The model under review builds one solid part; all positions refer to its coordinate system, in mm. Face numbers are marked on the shaded views. A direction names the side the tool comes from. Coordinates: 2 decimals unless noted, no trailing zeros. Order: outer loops, then holes, each group sorted by start corner. A loop starts at its lowest first (then second) coordinate and runs counter-clockwise, first axis right, second up. Notation, with made-up numbers: (-17, 74.25) -> (-11, 74.25) arc R18 cw to (-11, 92.25) -> close; hole circle Ø9 at (55, 6). An arc over 180 degrees is marked (long way). Put each result on its own line as item: value.
Autodesk Inventor part; units mm, degrees
ref_plane "XZ Plane" through (0, 0, 0) normal (0, 1, 0) x (-1, 0, 0)
sketch "Sketch1" plane through (0, 0, 0) normal (0, 1, 0) x (-1, 0, 0)
  line L0 (50.8, 50.8) -> (-50.8, 50.8)
  line L1 (-50.8, 50.8) -> (-50.8, -50.8)
  line L2 (-50.8, -50.8) -> (50.8, -50.8)
  line L3 (50.8, -50.8) -> (50.8, 50.8)
  line L4 (50.8, 50.8) -> (-50.8, -50.8) construction
  line L5 (-50.8, 50.8) -> (50.8, -50.8) construction
  point P0 (0, 0)
  dimension "d0" = 101.6
  dimension "d1" = 101.6
extrude "Extrusion1" add sketch "Sketch1" along normal blind 6.35
sketch "Sketch4" plane through (0, 6.35, 0) normal (0, 1, 0) x (1, 0, 0)
  line L0 (-25.4, -50.8) -> (25.4, -50.8)
  line L1 (25.4, -50.8) -> (25.4, 50.8)
  line L2 (25.4, 50.8) -> (-25.4, 50.8)
  line L3 (-25.4, 50.8) -> (-25.4, -50.8)
  line L4 (-25.4, -50.8) -> (25.4, 50.8) construction
  line L5 (25.4, -50.8) -> (-25.4, 50.8) construction
  line L6 (-50.8, 50.8) -> (-50.8, -50.8)
  line L7 (-50.8, -50.8) -> (50.8, -50.8)
  point P0 (0, 0)
  point P1 (0, 0)
  dimension "d15" = 50.8
  dimension "d16" = 25.4
  dimension "d17" = 101.6
extrude "Extrusion4" add sketch "Sketch4" along normal blind 59.6392
sketch "Sketch12" plane through (0, 65.9892, 0) normal (0, 1, 0) x (1, 0, 0)
  circle A0 centre (-12.7, -25.4) radius 2.5797
  line L0 (-25.4, -50.8) -> (25.4, -50.8)
  line L1 (-25.4, 50.8) -> (-25.4, -50.8)
  line L2 (-12.7, -25.4) -> (-12.7, 50.8) construction
  line L3 (-12.7, -25.4) -> (25.4, -25.4) construction
  circle A1 centre (-12.7, 0) radius 2.5797
  circle A2 centre (-12.7, 25.4) radius 2.5797
  circle A3 centre (12.7, -25.4) radius 2.5797
  circle A4 centre (12.7, 0) radius 2.5797
  circle A5 centre (12.7, 25.4) radius 2.5797
  point P0 (0, 0)
  dimension "d52" = 5.1594
  dimension "d53" = 25.4
  dimension "d54" = 12.7
  dimension "d57" = 25.4
  dimension "d60" = 25.4
extrude "Extrusion8" cut sketch "Sketch12" against normal through all
sketch "Sketch13" plane through (0, 6.35, 0) normal (0, 1, 0) x (1, 0, 0)
  circle A0 centre (-38.1, -25.4) radius 3.3782
  line L0 (-50.8, -50.8) -> (-25.4, -50.8)
  line L1 (-50.8, 50.8) -> (-50.8, -50.8)
  line L2 (-38.1, -25.4) -> (-38.1, 50.8) construction
  line L3 (-25.4, 50.8) -> (-50.8, 50.8)
  line L4 (-38.1, -25.4) -> (50.8, -25.4) construction
  line L5 (50.8, -50.8) -> (50.8, 50.8)
  line L6 (-38.1, 0) -> (50.8, 0) construction
  circle A1 centre (-38.1, 0) radius 3.3782
  line L7 (-38.1, 0) -> (-38.1, 76.2) construction
  line L8 (-38.1, 25.4) -> (50.8, 25.4) construction
  circle A2 centre (-38.1, 25.4) radius 3.3782
  line L9 (-38.1, 25.4) -> (-38.1, 101.6) construction
  line L10 (38.1, -25.4) -> (127, -25.4) construction
  circle A3 centre (38.1, -25.4) radius 3.3782
  line L11 (38.1, -25.4) -> (38.1, 50.8) construction
  line L12 (38.1, 0) -> (127, 0) construction
  circle A4 centre (38.1, 0) radius 3.3782
  line L13 (38.1, 0) -> (38.1, 76.2) construction
  line L14 (38.1, 25.4) -> (127, 25.4) construction
  circle A5 centre (38.1, 25.4) radius 3.3782
  line L15 (38.1, 25.4) -> (38.1, 101.6) construction
  point P0 (0, 0)
  dimension "d65" = 6.7564
  dimension "d66" = 25.4
  dimension "d67" = 12.7
  dimension "d70" = 25.4
  dimension "d73" = 76.2
extrude "Extrusion9" cut sketch "Sketch13" against normal through all
equation "\"d0\" = width"
equation "\"d1\" = length"
equation "\"d2\" = thickness"
equation "\"width\" = 101.6"
equation "\"length\" = 101.6"
equation "\"thickness\" = 6.35"
properties part number "SupportPlateMotorMountV01" material "Aluminum 6061"
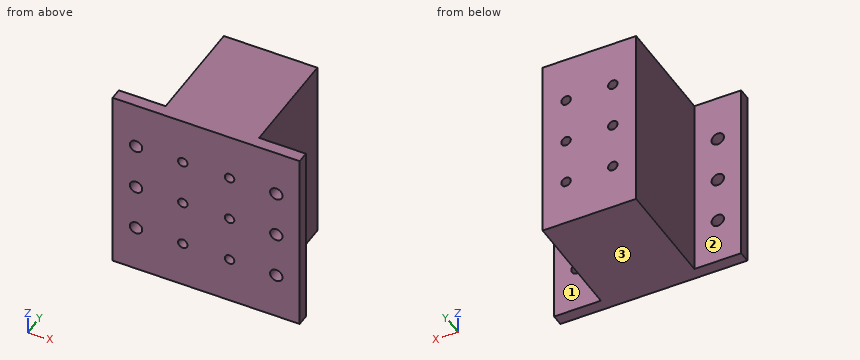
Item 1: Consider section C-C on y = 47.5. Write out the cut boundary in (x, z), and give its area (3 significant figures).
Answers below:
outline: (-25.4, -50.8) -> (25.4, -50.8) -> (25.4, 50.8) -> (-25.4, 50.8) -> close; hole circle Ø5.16 at (-12.7, -25.4); hole circle Ø5.16 at (-12.7, 0); hole circle Ø5.16 at (-12.7, 25.4); hole circle Ø5.16 at (12.7, -25.4); hole circle Ø5.16 at (12.7, 0); hole circle Ø5.16 at (12.7, 25.4)
area: 5,040 mm^2
Item 2: For line 1 (X direction, y = 3, z = 0); line 2 (X direction, y = 5, z = 25); line 3 (Z direction, x = 12.7, y = 28), list the stretches that pass through material, from the lowest coordinate up. Write a range as from..to.
Answers below:
line 1: -50.8..-41.48, -34.72..-15.28, -10.12..10.12, 15.28..34.72, 41.48..50.8
line 2: -50.8..-41.45, -34.75..-15.25, -10.15..10.15, 15.25..34.75, 41.45..50.8
line 3: -50.8..-27.98, -22.82..-2.58, 2.58..22.82, 27.98..50.8
Item 3: Consider section D-D on x = 38.1. Write out the cut boundary in (y, z), and give its area (3 significant figures).
Answers below:
outline: (0, -50.8) -> (6.35, -50.8) -> (6.35, -28.78) -> (0, -28.78) -> close; (0, -22.02) -> (6.35, -22.02) -> (6.35, -3.38) -> (0, -3.38) -> close; (0, 3.38) -> (6.35, 3.38) -> (6.35, 22.02) -> (0, 22.02) -> close; (0, 28.78) -> (6.35, 28.78) -> (6.35, 50.8) -> (0, 50.8) -> close
area: 516 mm^2
Item 4: Consider section A-A on x = -12.7. Write out the cut boundary in (y, z), and give its area (3 significant figures).
Answers below:
outline: (0, -50.8) -> (65.99, -50.8) -> (65.99, -27.98) -> (0, -27.98) -> close; (0, -22.82) -> (65.99, -22.82) -> (65.99, -2.58) -> (0, -2.58) -> close; (0, 2.58) -> (65.99, 2.58) -> (65.99, 22.82) -> (0, 22.82) -> close; (0, 27.98) -> (65.99, 27.98) -> (65.99, 50.8) -> (0, 50.8) -> close
area: 5,680 mm^2
Item 5: Consider section B-B on z = 25.4. Write out the cut boundary in (x, y).
Answers below:
outline: (-50.8, 0) -> (-41.48, 0) -> (-41.48, 6.35) -> (-50.8, 6.35) -> close; (-34.72, 0) -> (-15.28, 0) -> (-15.28, 65.99) -> (-25.4, 65.99) -> (-25.4, 6.35) -> (-34.72, 6.35) -> close; (-10.12, 0) -> (10.12, 0) -> (10.12, 65.99) -> (-10.12, 65.99) -> close; (15.28, 0) -> (34.72, 0) -> (34.72, 6.35) -> (25.4, 6.35) -> (25.4, 65.99) -> (15.28, 65.99) -> close; (41.48, 0) -> (50.8, 0) -> (50.8, 6.35) -> (41.48, 6.35) -> close
Item 6: For pin 1 Ø5 at (y, z) = (11, -34) entering from -X; pin 2 Ø1.5 at (y, z) = (8, -25) entering from +X; pin 3 Ø4.5 at (x, z) = (12.7, 0) entering from +Y, all flat-tipped, find the tip position at first contact; note any pin that passes through.
Answers below:
pin 1: x = -25.4
pin 2: x = 25.4
pin 3: through
Item 7: For the marked faces 1, 2 and 3, list the 3-axis set-ups (+Z, -Z, +X, -X, +Y, -Y) from which the entire face can be reached by the end or side of a thin tool; tool diameter is ignored.
Answers below:
face 1: +Z, -Z, +X, +Y
face 2: +Z, -Z, -X, +Y
face 3: -Z, +X, -X, +Y, -Y
